Could you check a few things on this model? Use its own coordinates, in mm. A direction names the side the tool comes from. Coordinates: 2 decimals unless noted, no trailing zeros. Write each loop counter-clockwise with the first axis right and the second up, starting at its lowest first coordinate (ties: lowest second). Pieces come first, ordered by that corner, then holes.
```python
from build123d import *

# Parameters (mm, degrees)
BOSS_EXTRU_1_DEPTH      = 170
ENL_V_MAT_EXTRU_1_DEPTH = 257.70995306


with BuildPart() as part:
    # Esquisse1 → Boss.-Extru.1 (new body)
    with BuildSketch(Plane.XY):
        Polygon((0, 90), (0, 0), (7, 0), (7, 80), (13, 80), (13, 0), (20, 0), (20, 20.562593983), (89.86150576, 80), (170, 80), (170, 90), align=None)
    extrude(amount=BOSS_EXTRU_1_DEPTH)

    # Esquisse3 → Enlèv. mat.-Extru.1 (cut, through all)
    with BuildSketch(Plane.XY.offset(170)):
        Polygon((20, 80), (79.058990958, 80), (20, 29.753255583), align=None)
    extrude(amount=-ENL_V_MAT_EXTRU_1_DEPTH, mode=Mode.SUBTRACT)


solid = part.part
```
Item 1: I want a section at C-C, the plane x = 45. List the corners of the cut face in (y, z) for me.
Item 2: Will these pins go through, and if not, where does the flat tip stop? pin 1 Ø25 at (y, z) = (62, 49) entering from +X; pin 2 Ø6.5 at (x, z) = (8.5, 111) entering from -Y; pin 3 Ø1 at (x, z) = (40.5, 23) entering from -Y; pin 4 Ø6 at (y, z) = (15, 58.5) entering from +X.
Item 3: If we mould it in two halves opening along Y, with no side actions, what happens to faces 1 (the flat face through (59, 62, 170)), 2 (the flat face through (49, 80, 86)), 3 (the flat face through (54.442, 49.865, 83.81)), 4 (the flat face through (86, 90, 84))? For each: released by +Y, released by -Y, zero draft, split by the parting line, or undercut.
Item 4: I want a section at A-A, the plane z = 144.5. List the corners of the cut face in (x, y) for me.
Item 5: If I drill on line 1 along X through (y, z) = (8, 71.5); line 2 along X through (y, z) = (53, 133.5); line 3 along X through (y, z) = (30.5, 106), over which ranges is the centre line in solid material (lowest first)?
Item 6: I want a section at B-B, the plane y = 66.5. List the corners of the cut face in (x, z) for me.
Item 7: I want a section at D-D, the plane x = 118. List the corners of the cut face in (y, z) for me.
Item 8: Which directions (+Z, -Z, +X, -X, +Y, -Y) give clear straight access to the entire face, cutting with the end or side of a thin tool? Please do faces 5 (the flat face through (0, 46, 84)), 6 (the flat face through (13, 41, 84)), 7 (the flat face through (59, 62, 0)), 8 (the flat face through (129, 80, 84)), 9 (the flat face through (49.943, 55.228, 86.19)).
Taken from the geometry:
1. outline: (41.83, 0) - (51.02, 0) - (51.02, 170) - (41.83, 170) - close; (80, 0) - (90, 0) - (90, 170) - (80, 170) - close
2. pin 1: stops at x = 83.4
2. pin 2: stops at y = 0
2. pin 3: stops at y = 37.58
2. pin 4: stops at x = 20
3. face 1: zero draft
3. face 2: undercut
3. face 3: released by -Y
3. face 4: released by +Y
4. outline: (0, 0) - (7, 0) - (7, 80) - (13, 80) - (13, 0) - (20, 0) - (20, 20.56) - (89.86, 80) - (170, 80) - (170, 90) - (0, 90) - close; hole (20, 29.75) - (79.06, 80) - (20, 80) - close
5. line 1: x = 0 to 7, 13 to 20
5. line 2: x = 0 to 7, 13 to 20, 47.32 to 58.13
5. line 3: x = 0 to 7, 13 to 20, 20.88 to 31.68
6. outline: (0, 0) - (7, 0) - (7, 170) - (0, 170) - close; (13, 0) - (20, 0) - (20, 170) - (13, 170) - close; (63.19, 0) - (73.99, 0) - (73.99, 170) - (63.19, 170) - close
7. outline: (80, 0) - (90, 0) - (90, 170) - (80, 170) - close
8. face 5: +Z, -Z, -X, +Y, -Y
8. face 6: +Z, -Z, -Y
8. face 7: -Z, +X, -X, +Y, -Y
8. face 8: +Z, -Z, +X, -Y
8. face 9: +Z, -Z
